The model under review builds one solid part; all positions refer to its coordinate system, in mm. A direction names the side the tool comes from. Coordinates: 2 decimals unless noted, no trailing zeros. Order: outer loops, then holes, each group sorted by start corner. A loop starts at its lowest first (then second) coordinate and runs counter-clockwise, first axis right, second up. Notation, with made-up numbers: (57.5, -13.75) -> (80.5, -13.75) arc R31 ccw to (80.5, 22.25) -> close; hole circle Ø10 at (24.5, 77). An arc over 180 degrees is marked (long way). Put each result on its own line as item: value.
from build123d import *

# Parameters (mm, degrees)
SKETCH1_W                                    = 60
SKETCH1_H                                    = 45
BOSS_EXTRUDE1_DEPTH                          = 10
SKETCH2_W                                    = 40.5
SKETCH2_H                                    = 40.5
CUT_EXTRUDE1_DEPTH                           = 4
SKETCH3_R                                    = 20
CUT_EXTRUDE2_DEPTH                           = 10
FILLET1_R                                    = 1
F_2_8_2_8_DIAMETER_HOLE1_D                   = 2.8
F_2_8_2_8_DIAMETER_HOLE1_CSINK_D             = 2.85
F_2_8_2_8_DIAMETER_HOLE1_CSINK_ANGLE         = 90
CBORE_FOR_M3_HEX_SOCKET_HEAD_CAP_SCR_2_COUNT = 2
CBORE_FOR_M3_HEX_SOCKET_HEAD_CAP_SCR_2_PITCH = 30.516389039
CBORE_FOR_M3_HEX_SOCKET_HEAD_CAP_SCR_3_COUNT = 2
CBORE_FOR_M3_HEX_SOCKET_HEAD_CAP_SCR_3_PITCH = 61.032778079
CBORE_FOR_M3_HEX_SOCKET_HEAD_CAP_SCR_4_COUNT = 2
CBORE_FOR_M3_HEX_SOCKET_HEAD_CAP_SCR_4_PITCH = 50
CBORE_FOR_M3_HEX_SOCKET_HEAD_CAP_SCR_5_COUNT = 2
CBORE_FOR_M3_HEX_SOCKET_HEAD_CAP_SCR_5_PITCH = 35
FILLET3_R                                    = 2


with BuildPart() as part:
    # Sketch1 → Boss-Extrude1 (new body)
    with BuildSketch(Plane(origin=(0, 0, 0), x_dir=(0, 0, -1), z_dir=(1, 0, 0))):
        Rectangle(SKETCH1_W, SKETCH1_H)
    extrude(amount=BOSS_EXTRUDE1_DEPTH)

    # Sketch2 → Cut-Extrude1 (cut)
    with BuildSketch(Plane(origin=(10, 0, 0), x_dir=(0, 0, -1), z_dir=(1, 0, 0))):
        Rectangle(SKETCH2_W, SKETCH2_H)
    extrude(amount=-CUT_EXTRUDE1_DEPTH, mode=Mode.SUBTRACT)

    # Sketch3 → Cut-Extrude2 (cut)
    with BuildSketch(Plane(origin=(6, 0, 0), x_dir=(0, 0, -1), z_dir=(1, 0, 0))):
        Circle(SKETCH3_R)
    extrude(amount=-CUT_EXTRUDE2_DEPTH, mode=Mode.SUBTRACT)

    # Fillet1
    fillet1_edges = [part.edges().sort_by_distance(p)[0] for p in [
        (8, 20.25, -20.25),
        (8, -20.25, -20.25),
        (8, -20.25, 20.25),
        (8, 20.25, 20.25),
    ]]
    fillet(fillet1_edges, radius=FILLET1_R)

    # Ø2.8 (2.8) Diameter Hole1 (through all)
    with Locations(Plane(origin=(6, 0, 0), x_dir=(0, 0, -1), z_dir=(1, 0, 0))):
        with Locations((0, 0), (16, -16), (-16, 16), (-16, -16), (16, 16)):
            CounterSinkHole(F_2_8_2_8_DIAMETER_HOLE1_D / 2, F_2_8_2_8_DIAMETER_HOLE1_CSINK_D / 2, counter_sink_angle=F_2_8_2_8_DIAMETER_HOLE1_CSINK_ANGLE)

    # Sketch14 → CBORE for M3 Hex Socket Head Cap Screw2 (revolve, cut)
    with BuildSketch(Plane(origin=(10, -17.5, -25), x_dir=(0, 0, -1), z_dir=(0, 1, 0))):
        Polygon((0, 0), (0, 10), (1.7, 10), (1.7, 3.4), (3.25, 3.4), (3.25, 0.025), (3.275, 0), align=None)
    cbore_for_m3_hex_socket_head_cap_screw2 = revolve(axis=Axis((16.35, -17.5, -25), (-1, 0, 0)), mode=Mode.SUBTRACT)

    # CBORE for M3 Hex Socket Head Cap Scr 2: CBORE for M3 Hex Socket Head Cap Screw2 ×2
    with Locations(*[Vector(0, 0.5734623443633283, 0.8192319205190406) * (i * CBORE_FOR_M3_HEX_SOCKET_HEAD_CAP_SCR_2_PITCH) for i in range(1, CBORE_FOR_M3_HEX_SOCKET_HEAD_CAP_SCR_2_COUNT)]):
        add(cbore_for_m3_hex_socket_head_cap_screw2, mode=Mode.SUBTRACT)

    # CBORE for M3 Hex Socket Head Cap Scr 3: CBORE for M3 Hex Socket Head Cap Screw2 ×2
    with Locations(*[Vector(0, 0.5734623443633283, 0.8192319205190406) * (i * CBORE_FOR_M3_HEX_SOCKET_HEAD_CAP_SCR_3_PITCH) for i in range(1, CBORE_FOR_M3_HEX_SOCKET_HEAD_CAP_SCR_3_COUNT)]):
        add(cbore_for_m3_hex_socket_head_cap_screw2, mode=Mode.SUBTRACT)

    # CBORE for M3 Hex Socket Head Cap Scr 4: CBORE for M3 Hex Socket Head Cap Screw2 ×2
    with Locations(*[(0, 0, i * CBORE_FOR_M3_HEX_SOCKET_HEAD_CAP_SCR_4_PITCH) for i in range(1, CBORE_FOR_M3_HEX_SOCKET_HEAD_CAP_SCR_4_COUNT)]):
        add(cbore_for_m3_hex_socket_head_cap_screw2, mode=Mode.SUBTRACT)

    # CBORE for M3 Hex Socket Head Cap Scr 5: CBORE for M3 Hex Socket Head Cap Screw2 ×2
    with Locations(*[(0, i * CBORE_FOR_M3_HEX_SOCKET_HEAD_CAP_SCR_5_PITCH, 0) for i in range(1, CBORE_FOR_M3_HEX_SOCKET_HEAD_CAP_SCR_5_COUNT)]):
        add(cbore_for_m3_hex_socket_head_cap_screw2, mode=Mode.SUBTRACT)

    # Fillet3
    fillet3_edges = [part.edges().sort_by_distance(p)[0] for p in [
        (5, -22.5, -30),
        (5, -22.5, 30),
        (5, 22.5, 30),
        (5, 22.5, -30),
    ]]
    fillet(fillet3_edges, radius=FILLET3_R)


solid = part.part
Item 1: For line 1 (Y direction, x = 3, z = -25); line 2 (Z direction, x = 7.95, y = -17.5); line 3 (Y direction, x = 8.65, z = 25), list the stretches that pass through material, from the lowest coordinate up. Write a range as from..to.
Answers below:
line 1: -22.5..-19.2, -15.8..15.8, 19.2..22.5
line 2: -30..-28.25, -21.75..-20.25, 20.25..21.75, 28.25..30
line 3: -22.5..-20.75, -14.25..14.25, 20.75..22.5
Item 2: Mouldability with a two-part tool opening along Y and no side actions: class faces 1 (the cylindrical face through (3.35, 16.99, -26.62)), 2 (the cylindrical face through (5.07, -21.93, -29.4)), 3 (the flat face through (0, 15, 14)) as +Y half, -Y half, draft (parallel to the pull), parting line (faces both ways), or undercut.
Answers below:
face 1: undercut
face 2: -Y half
face 3: draft
Item 3: For pin 1 Ø4 at (y, z) = (17.5, 25) entering from +X, flat-tipped, find the tip position at first contact; note if it passes through.
Answers below:
pin 1: x = 6.6
Item 4: Consider section C-C on z = -25. Write out the cut boundary in (x, y) (3 decimals).
Answers below:
outline: (0, -22.5) -> (10, -22.5) -> (10, -20.775) -> (9.975, -20.75) -> (6.6, -20.75) -> (6.6, -19.2) -> (0, -19.2) -> close; (0, -15.8) -> (6.6, -15.8) -> (6.6, -14.25) -> (9.975, -14.25) -> (10, -14.225) -> (10, 14.225) -> (9.975, 14.25) -> (6.6, 14.25) -> (6.6, 15.8) -> (0, 15.8) -> close; (0, 19.2) -> (6.6, 19.2) -> (6.6, 20.75) -> (9.975, 20.75) -> (10, 20.775) -> (10, 22.5) -> (0, 22.5) -> close
Item 5: Consider section B-B on y = 0. Write out the cut boundary in (x, z).
Answers below:
outline: (0, -30) -> (10, -30) -> (10, -20.25) -> (6, -20.25) -> (6, -20) -> (0, -20) -> close; (0, 20) -> (6, 20) -> (6, 20.25) -> (10, 20.25) -> (10, 30) -> (0, 30) -> close
Item 6: For faces 4 (the flat face through (5, -22.5, 0)), 5 (the flat face through (6, -4, 20)), list the 3-axis set-ups (+Z, -Z, +X, -X, +Y, -Y) from which the entire face can be reached by the end or side of a thin tool; tool diameter is ignored.
Answers below:
face 4: +Z, -Z, +X, -X, -Y
face 5: +X
Item 7: Consider section D-D on z = 16. Write out the cut boundary in (x, y) (3 decimals), and give its area (3 significant figures).
Answers below:
outline: (0, -22.5) -> (10, -22.5) -> (10, -20.25) -> (6, -20.25) -> (6, -17.425) -> (5.975, -17.4) -> (0, -17.4) -> close; (0, -14.6) -> (5.975, -14.6) -> (6, -14.575) -> (6, -12) -> (0, -12) -> close; (0, 12) -> (6, 12) -> (6, 14.575) -> (5.975, 14.6) -> (0, 14.6) -> close; (0, 17.4) -> (5.975, 17.4) -> (6, 17.425) -> (6, 20.25) -> (10, 20.25) -> (10, 22.5) -> (0, 22.5) -> close
area: 110 mm^2
Item 8: Consider section A-A on z = 0. Write out the cut boundary in (x, y), and give its area (3 significant figures).
Answers below:
outline: (0, -22.5) -> (10, -22.5) -> (10, -20.25) -> (6, -20.25) -> (6, -20) -> (0, -20) -> close; (0, 20) -> (6, 20) -> (6, 20.25) -> (10, 20.25) -> (10, 22.5) -> (0, 22.5) -> close
area: 48.0 mm^2
